```python
from build123d import *

# Parameters (mm, degrees)
SKETCH1_W           = 18
SKETCH1_H           = 70.5
BOSS_EXTRUDE1_DEPTH = 0.6
SKETCH3_R           = 1.3
CUT_EXTRUDE1_DEPTH  = 10
SKETCH4_W           = 1
SKETCH4_H           = 64.56
BOSS_EXTRUDE2_DEPTH = 1.5


with BuildPart() as part:
    # Sketch1 → Boss-Extrude1 (new body)
    with BuildSketch(Plane(origin=(0, 0, 0), x_dir=(1, 0, 0), z_dir=(0, 1, 0))):
        with Locations((9, 35.25)):
            Rectangle(SKETCH1_W, SKETCH1_H)
    extrude(amount=BOSS_EXTRUDE1_DEPTH)

    # Sketch3 → Cut-Extrude1 (cut)
    with BuildSketch(Plane(origin=(0, 0.6, 0), x_dir=(1, 0, 0), z_dir=(0, 1, 0))):
        with Locations((10.9, 10.48)):
            Circle(SKETCH3_R)
        with Locations((10.9, 32.83)):
            Circle(SKETCH3_R)
        with Locations((10.9, 55.18)):
            Circle(SKETCH3_R)
    extrude(amount=-CUT_EXTRUDE1_DEPTH, mode=Mode.SUBTRACT)

    # Sketch4 → Boss-Extrude2 (add)
    with BuildSketch(Plane.XZ):
        with Locations((5.15, -32.28)):
            Rectangle(SKETCH4_W, SKETCH4_H)
        with Locations((16.65, -32.28)):
            Rectangle(SKETCH4_W, SKETCH4_H)
    extrude(amount=BOSS_EXTRUDE2_DEPTH)


solid = part.part
```
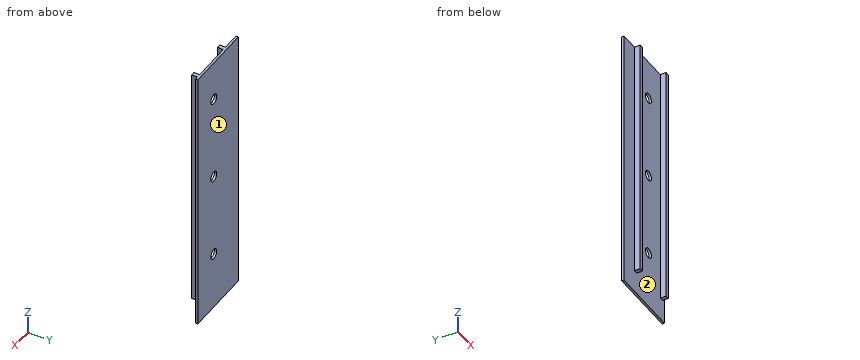
Read the model definition and answer for the solid it produces. Units are mm, in the model's axes. Face numbers are marked on the shaded views. Coordinates: 2 decimals unless noted, no trailing zeros. Write each loop counter-clockwise with the first axis right and the second up, starting at its lowest first coordinate (ties: lowest second). Pieces come first, ordered by that corner, then holes. Notation, with made-up numbers: (-22, -38.75) -> (36, -38.75) arc R18 cw to (36, -11.75) -> close; hole circle Ø3 at (26.25, 9.5). An arc over 180 degrees is marked (long way). Return JSON: item names as keys, results as strings.
1. Each of these flat-tipped pins is pushed along its axis until it touches: P1, Ø3.5, axis at x = 10.9, z = -10.48, coming from the -Y side; P2, Ø0.8, axis at y = -1, z = -42.5, coming from the +X side; P3, Ø1.6, axis at x = 10.9, z = -32.83, coming from the -Y side; P4, Ø1.2, axis at y = -1, z = -36, coming from the -X side. Where does it stop, or does it pass through?
Found:
{"P1": "y = 0", "P2": "x = 17.15", "P3": "through", "P4": "x = 4.65"}
2. A cutting plane is placed at D-D (z = -49). Determine the outline of the cut face in (x, y), and give its area (3 significant figures).
Found:
{"outline": "(0, 0) -> (4.65, 0) -> (4.65, -1.5) -> (5.65, -1.5) -> (5.65, 0) -> (16.15, 0) -> (16.15, -1.5) -> (17.15, -1.5) -> (17.15, 0) -> (18, 0) -> (18, 0.6) -> (0, 0.6) -> close", "area": "13.8 mm2"}
3. A cutting plane is placed at B-B (z = -32.83). Determine the outline of the cut face in (x, y).
Found:
{"outline": "(0, 0) -> (4.65, 0) -> (4.65, -1.5) -> (5.65, -1.5) -> (5.65, 0) -> (9.6, 0) -> (9.6, 0.6) -> (0, 0.6) -> close; (12.2, 0) -> (16.15, 0) -> (16.15, -1.5) -> (17.15, -1.5) -> (17.15, 0) -> (18, 0) -> (18, 0.6) -> (12.2, 0.6) -> close"}
4. Find the intervals of material crossed by line 1 along Z through (x, y) = (10.9, 0.2); line 2 along X through (y, z) = (-0.45, -57.5); line 3 along X through (y, z) = (0.35, -32.83), in increasing order. Write a range as from..to.
Found:
{"line 1": "-70.5..-56.48, -53.88..-34.13, -31.53..-11.78, -9.18..0", "line 2": "4.65..5.65, 16.15..17.15", "line 3": "0..9.6, 12.2..18"}
5. A cutting plane is placed at A-A (x = 10.9). Determine the outline of the cut face in (y, z), and give its area (3 significant figures).
Found:
{"outline": "(0, -70.5) -> (0.6, -70.5) -> (0.6, -56.48) -> (0, -56.48) -> close; (0, -53.88) -> (0.6, -53.88) -> (0.6, -34.13) -> (0, -34.13) -> close; (0, -31.53) -> (0.6, -31.53) -> (0.6, -11.78) -> (0, -11.78) -> close; (0, -9.18) -> (0.6, -9.18) -> (0.6, 0) -> (0, 0) -> close", "area": "37.6 mm2"}
6. A cutting plane is placed at C-C (y = -0.5). Determine the outline of the cut face in (x, z).
Found:
{"outline": "(4.65, -64.56) -> (5.65, -64.56) -> (5.65, 0) -> (4.65, 0) -> close; (16.15, -64.56) -> (17.15, -64.56) -> (17.15, 0) -> (16.15, 0) -> close"}
7. Determine the mould class of the marked faces 1 and 2 for opening direction X: pulls with the +X half, pulls with the -X half, needs draft (parallel to the pull), parting line crosses it, or undercut.
Found:
{"face 1": "needs draft", "face 2": "undercut"}
